Verification items for this drawing (mm, ordinates from the low corner). A direction names the side the tool comes from. Round coordinates to 2 decimals unless told otherwise and drop trailing zeros. Loops run counter-clockwise (first coordinate to the right, second up) from the corner with the lowest first, then second, coordinate; pieces in that order, holes last. Notation, with made-up numbers: (3, 40) - (28, 40) arc R9 ccw to (28, 55) - close; hole circle Ø5 at (84, 61.25). An arc over 180 degrees is marked (long way). Put each result on its own line as item: value.
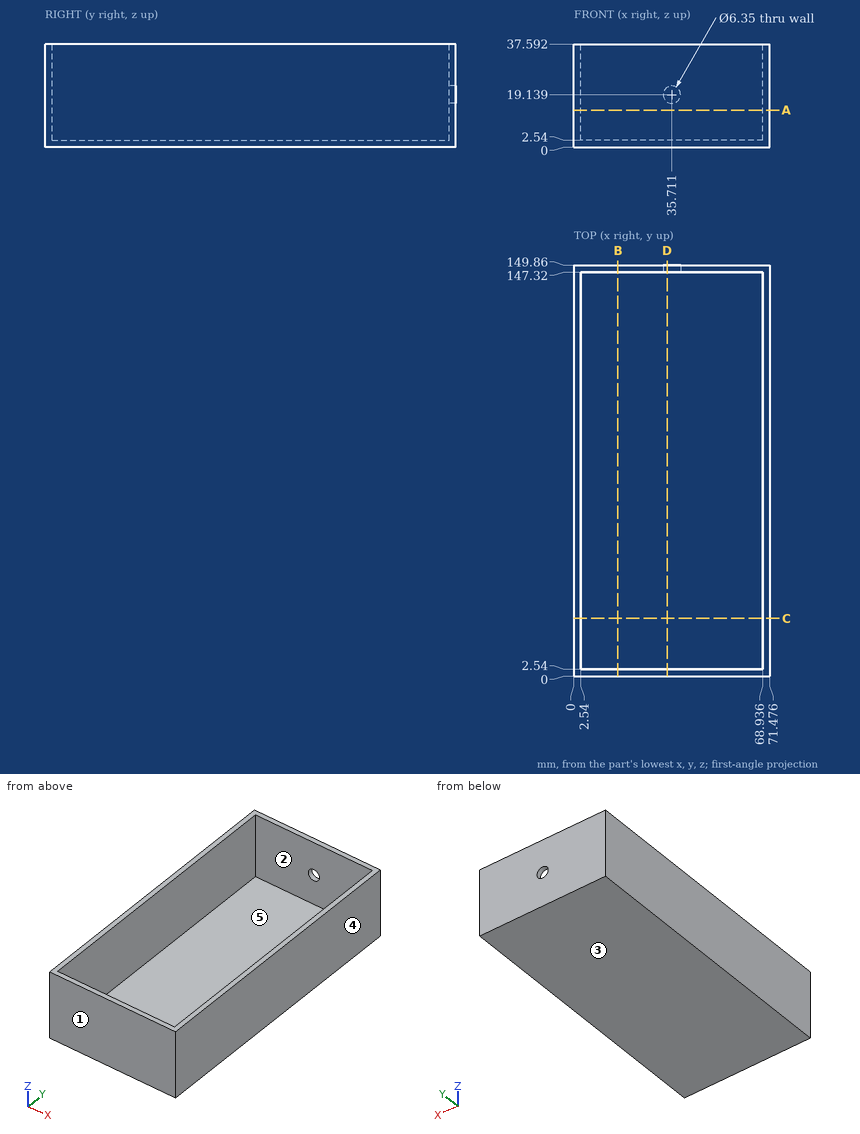
Item 1: Thickness scan on line 1 (X direction, y = 56, z = 22) (1 decimal); line 2 (Y direction, x = 31, z = 24.5); line 3 (Z direction, x = 66.5, y = 137). Record the ranges inside material, lowest first. Write a range as from..to.
Filled sheet:
line 1: 0..2.5, 68.9..71.5
line 2: 0..2.54, 147.32..149.86
line 3: 0..2.54
Item 2: Go/stop test with a flat-tipped pin: pin 1 (6 mm diameter, centred on x = 62.5, y = 66, fed in from +Z). Record where the tip stops, or that it passes through.
Filled sheet:
pin 1: z = 2.54
Item 3: Section check A-A on z = 13.5. Enter the section's corners in (x, y) (1 decimal), then the cut area to 3 significant figures.
Filled sheet:
outline: (0, 0) - (71.5, 0) - (71.5, 149.9) - (0, 149.9) - close; hole (2.5, 2.5) - (68.9, 2.5) - (68.9, 147.3) - (2.5, 147.3) - close
area: 1,100 mm²
Item 4: Section check C-C on y = 21. Enter the section's corners in (x, z) (1 decimal).
Filled sheet:
outline: (0, 0) - (71.5, 0) - (71.5, 37.6) - (68.9, 37.6) - (68.9, 2.5) - (2.5, 2.5) - (2.5, 37.6) - (0, 37.6) - close
Item 5: Section check D-D on x = 34. Enter the section's corners in (y, z) (1 decimal), then the cut area to 3 significant figures.
Filled sheet:
outline: (0, 0) - (149.9, 0) - (149.9, 16.5) - (147.3, 16.5) - (147.3, 2.5) - (2.5, 2.5) - (2.5, 37.6) - (0, 37.6) - close; (147.3, 21.8) - (149.9, 21.8) - (149.9, 37.6) - (147.3, 37.6) - close
area: 545 mm²
Item 6: Section check B-B on x = 16. Enter the section's corners in (y, z).
Filled sheet:
outline: (0, 0) - (149.86, 0) - (149.86, 37.59) - (147.32, 37.59) - (147.32, 2.54) - (2.54, 2.54) - (2.54, 37.59) - (0, 37.59) - close
Item 7: Tool access check on the marked faces 4 and 5. Record the directions out of +Z, -Z, +X, -X, +Y, -Y that give a thin tool (end or side, any length) a straight path to the whole face; none if there is none.
Filled sheet:
face 4: +Z, -Z, +X, +Y, -Y
face 5: +Z
Item 8: Release check for a two-part mould opening along Y. For the marked faces 1, 2 and 3 record: +Y half, -Y half, draft (parallel to the pull), parting line (faces both ways), or undercut.
Filled sheet:
face 1: -Y half
face 2: undercut
face 3: draft
